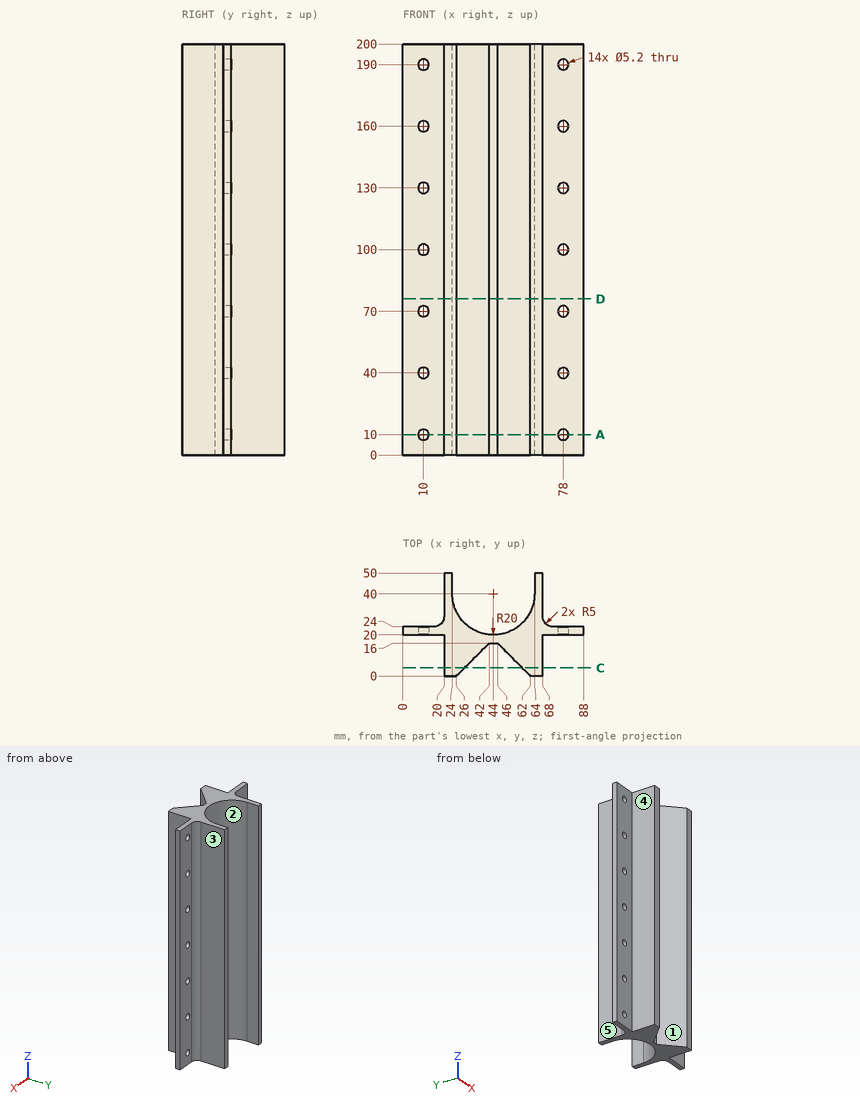
Geometry: see drawing. Coordinates: mm, zero at the bounding-box minimum. A direction names the side the tool comes from. Give positions to 0.01 mm unless a question says otherwise; leave off trailing zeros. Write each loop counter-clockwise with the first axis right and the second up, starting at its lowest first coordinate (ties: lowest second). Pieces come first, ordered by that corner, then holes. Notation, with made-up numbers: M -30,-9.5 L -3,-9.5 A16 ccw -3,0.5 Z; hole C -32,-3.75 d5. An arc over 180 degrees is marked long. Return JSON: item names as keys, results as strings. Group by question number.
1) Cut plane D-D, the plane z = 76. Output: boundary loops of the cut face in (x, y), then the cut area to 3 significant figures.
2) First-contact query: pin 1 Ø1.5 at (x, z) = (78.5, 146.5) entering from -Y; pin 2 Ø1.5 at (y, z) = (38, 143) entering from -X; pin 3 Ø16.5 at (x, z) = (78, 78.5) entering from +Y. Flat tips, straight axial feed; report the tip coordinate or a pass-through.
3) Ray query, L1, parallel to X at y = 42, z = 52; L2, parallel to X at y = 22.6, z = 130; L3, parallel to X at y = 22.95, z = 160. Return the intervals inside material, ascending.
4) Set-up query: the marked faces 1, 2, 3, 4 and 5. Return all of +Z, -Z, +X, -X, +Y, -Y with unobstructed straight access to the full face (end or side cutting, diameter ignored); none if empty.
5) Cut plane A-A, the plane z = 10. Give the number of separate pieces and of enclosed holes in the cut face, then the cut area to 3 significant figures.
6) Cut plane C-C, the plane y = 4. Output: boundary loops of the cut face in (x, z), then the cut area to 3 significant figures.
Data:
{
 "1": {"outline": "M 0,20 L 20,20 L 20,0 L 26,0 L 42,16 L 46,16 L 62,0 L 68,0 L 68,20 L 88,20 L 88,24 L 73,24 A5 cw 68,29 L 68,50 L 64,50 L 64,40 A20 cw 24,40 L 24,50 L 20,50 L 20,29 A5 cw 15,24 L 0,24 Z", "area": "1,220 mm²"},
 "2": {"pin 1": "stops at y = 20", "pin 2": "stops at x = 20", "pin 3": "stops at y = 25.2"},
 "3": {"L1": "x = 20 to 24, 64 to 68", "L2": "x = 0 to 7.4, 12.6 to 34.14, 53.86 to 75.4, 80.6 to 88", "L3": "x = 0 to 7.4, 12.6 to 33.55, 54.45 to 75.4, 80.6 to 88"},
 "4": {"face 1": "+Z, -Z, -Y", "face 2": "+Z, -Z, +Y", "face 3": "+Z, -Z, +X, +Y", "face 4": "+Z, -Z, -X, -Y", "face 5": "+Z, -Z, -X, +Y"},
 "5": {"separate pieces": "3", "enclosed holes": "0", "area": "1,180 mm²"},
 "6": {"outline": "M 20,0 L 30,0 L 30,200 L 20,200 Z; M 58,0 L 68,0 L 68,200 L 58,200 Z", "area": "4,000 mm²"}
}
